For this review, take the finished solid that the model builds, in its own axes (mm). Give positions to 0.01 mm unless a question says otherwise; leave off trailing zeros. Loops run counter-clockwise (first coordinate to the right, second up) from the corner with the lowest first, then second, coordinate; pieces in that order, holes last. Notation, with made-up numbers: (28, -13.75) - (55, -13.75) arc R31 ccw to (55, 16.25) - close; hole circle Ø2 at (16, 66). An arc over 180 degrees is marked (long way). Answer as CSV lines item,"result".
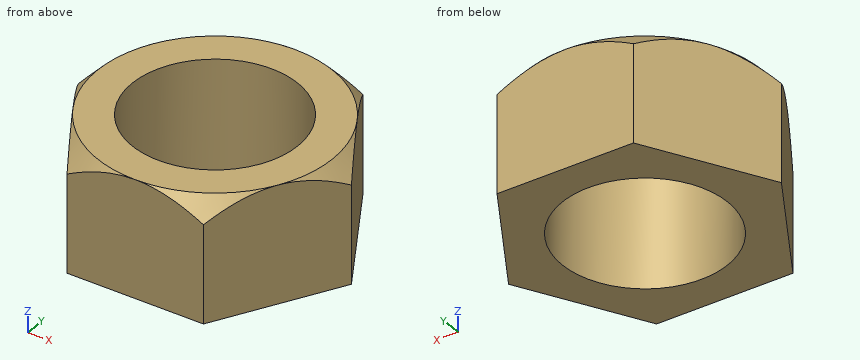
from build123d import *

# Parameters (mm, degrees)
CROQUIS1_R              = 6.35
SALIENTE_EXTRUIR1_DEPTH = 9
CROQUIS2_R              = 17.950209201
CROQUIS2_R_2            = 9
CORTAR_EXTRUIR1_DEPTH   = 9
CORTAR_EXTRUIR1_TAPER   = 43


with BuildPart() as part:
    # Croquis1 → Saliente-Extruir1 (new body)
    with BuildSketch(Plane.XY):
        Polygon((-10.392304845, 0), (-5.196152423, -9), (5.196152423, -9), (10.392304845, 0), (5.196152423, 9), (-5.196152423, 9), align=None)
        Circle(CROQUIS1_R, mode=Mode.SUBTRACT)
    extrude(amount=SALIENTE_EXTRUIR1_DEPTH)

    # Croquis2 → Cortar-Extruir1 (cut)
    with BuildSketch(Plane.XY.offset(9)):
        with Locations((-0.193993057, 0)):
            Circle(CROQUIS2_R)
        Circle(CROQUIS2_R_2, mode=Mode.SUBTRACT)
    extrude(amount=-CORTAR_EXTRUIR1_DEPTH, taper=CORTAR_EXTRUIR1_TAPER, mode=Mode.SUBTRACT)


solid = part.part
1) Insertion check: P1, Ø2, axis at y = -3.5, z = 2.5, coming from the -X side. The pin has a flat end and moves straight along its axis. Give the tip position at first contact, or say it passes through.
From the geometry:
P1,"stops at x = -8.95"
2) Wall thickness on line 1 (Y direction, x = 0, z = 6); line 2 (Y direction, x = -3, z = 2.5); line 3 (Z direction, x = -5, y = -7.75): over which ranges is each line inside the solid? List them lowest first. Write a range as from..to.
From the geometry:
line 1,"y = -9..-6.35, 6.35..9"
line 2,"y = -9..-5.6, 5.6..9"
line 3,"z = 0..8.76"
3) Consider section A-A on z = 4.75. Write out the cut boundary in (x, y).
From the geometry:
outline,"(-10.39, 0) - (-5.2, -9) - (5.2, -9) - (10.39, 0) - (5.2, 9) - (-5.2, 9) - close; hole circle Ø12.7 at (0, 0)"
4) Consider section B-B on z = 7.75. Write out the cut boundary in (x, y).
From the geometry:
outline,"(-10.16, -0.41) - (-5.43, -8.59) arc R10.17 ccw to (-4.73, -9) - (4.73, -9) arc R10.17 ccw to (5.43, -8.59) - (10.16, -0.41) arc R10.17 ccw to (10.16, 0.41) - (5.43, 8.59) arc R10.17 ccw to (4.73, 9) - (-4.73, 9) arc R10.17 ccw to (-5.43, 8.59) - (-10.16, 0.41) arc R10.17 ccw to start; hole circle Ø12.7 at (0, 0)"
